```python
from build123d import *

# Parameters (mm, degrees)
F0_W     = 362
F0_H     = 586
F0_R     = 37
F0_R_2   = 40
F1_DEPTH = 19
F2_DEPTH = 150
F0_R_3   = 34
F3_DEPTH = 150


with BuildPart() as f1:
    # F0 (on Front) → F1 (new body)
    with BuildSketch(Plane.XZ):
        with Locations((181, 293)):
            Rectangle(F0_W, F0_H)
        with Locations((100, 100)):
            Circle(F0_R, mode=Mode.SUBTRACT)
        with Locations((262, 100)):
            Circle(F0_R_2, mode=Mode.SUBTRACT)
    extrude(amount=F1_DEPTH)

    # F0 (on Front) → F2 (join)
    with BuildSketch(Plane.XZ):
        with Locations((262, 100)):
            Circle(F0_R_2)
        with Locations((262, 100)):
            Circle(F0_R, mode=Mode.SUBTRACT)
    extrude(amount=F2_DEPTH)

    # F0 (on Front) → F3 (join)
    with BuildSketch(Plane.XZ):
        with Locations((100, 100)):
            Circle(F0_R)
        with Locations((100, 100)):
            Circle(F0_R_3, mode=Mode.SUBTRACT)
    extrude(amount=F3_DEPTH)


solid = f1.part
```
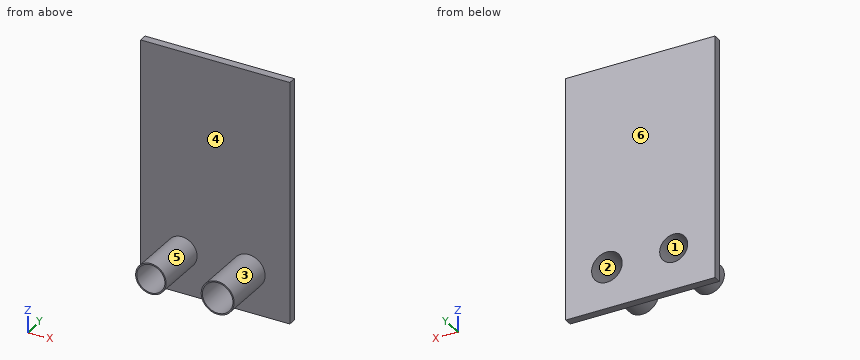
Model file for the job. Use its own axes, mm. Face numbers are marked on the shaded views. A direction names the side the tool comes from. Round coordinates to 2 decimals unless told otherwise and drop trailing zeros. Write each loop counter-clockwise with the first axis right and the second up, starting at its lowest first coordinate (ties: lowest second). Pieces come first, ordered by that corner, then holes. Notation, with made-up numbers: (74, 33.25) -> (102, 33.25) arc R23 cw to (102, 62.25) -> close; hole circle Ø8 at (13, 79.5). An arc over 180 degrees is marked (long way). Answer as CSV lines item,"result".
1. Pin check, flat tips, straight feed: pin 1 Ø8 at (x, y) = (237.5, -32.5) entering from -Z; pin 2 Ø12 at (x, y) = (131, -33) entering from -Z; pin 3 Ø10 at (x, y) = (230, -114) entering from -Z. Stop position of each tip, or through.
Resolved:
pin 1,"z = 65.65"
pin 2,"z = 72.72"
pin 3,"z = 70.49"
2. Tool access for the marked faces 5 and 6: list every direction of +Z, -Z, +X, -X, +Y, -Y with a clear straight run to the whole face (end or side of a thin tool).
Resolved:
face 5,"-Y"
face 6,"+Z, -Z, +X, -X, +Y"
3. Drill centre lines: line 1 (Z direction, x = 97.5, y = -83.5); line 2 (Z direction, x = 100, y = -66); line 3 (Y direction, x = 115, z = 473). Where is each one in solid material? Low to high.
Resolved:
line 1,"63.08 to 66.09, 133.91 to 136.92"
line 2,"63 to 66, 134 to 137"
line 3,"-19 to 0"
4. Slice it at B-B, the plane z = 100. List the corners of the cut face in (x, y), plus the area to 3 significant figures.
Resolved:
outline,"(0, -19) -> (63, -19) -> (63, -150) -> (66, -150) -> (66, 0) -> (0, 0) -> close; (134, -150) -> (137, -150) -> (137, -19) -> (222, -19) -> (222, -150) -> (225, -150) -> (225, 0) -> (134, 0) -> close; (299, -150) -> (302, -150) -> (302, -19) -> (362, -19) -> (362, 0) -> (299, 0) -> close"
area,"5,750 mm²"
5. Slice it at A-A, the plane x = 262. List the corners of the cut face in (y, z), plus the area to 3 significant figures.
Resolved:
outline,"(-150, 60) -> (-19, 60) -> (-19, 0) -> (0, 0) -> (0, 63) -> (-150, 63) -> close; (-150, 137) -> (0, 137) -> (0, 586) -> (-19, 586) -> (-19, 140) -> (-150, 140) -> close"
area,"10,500 mm²"
6. Slice it at D-D, the plane x = 100. List the corners of the cut face in (y, z).
Resolved:
outline,"(-150, 63) -> (-19, 63) -> (-19, 0) -> (0, 0) -> (0, 66) -> (-150, 66) -> close; (-150, 134) -> (0, 134) -> (0, 586) -> (-19, 586) -> (-19, 137) -> (-150, 137) -> close"
7. Mould opens along Z. For the marked faces 1, 2, 3 and 4 say: +Z half, -Z half, draft (parallel to the pull), parting line (faces both ways), or undercut.
Resolved:
face 1,"undercut"
face 2,"undercut"
face 3,"parting line"
face 4,"draft"
8. Slice it at C-C, the plane y = -130. List the corners of the cut face in (x, z), plus the area to 3 significant figures.
Resolved:
outline,"circle Ø74 at (100, 100); circle Ø80 at (262, 100); hole circle Ø68 at (100, 100); hole circle Ø74 at (262, 100)"
area,"1,390 mm²"
